The listing builds one solid part. Answer for the finished solid, in the listing's coordinates (mm). Give positions to 0.01 mm unless a question says otherwise; leave off trailing zeros. Write each loop counter-clockwise with the first axis right and the second up, starting at its lowest first coordinate (ties: lowest second). Pieces come first, ordered by that corner, then holes. Notation, with made-up numbers: M -31,22 L -6,22 A23 ccw -6,47 Z; hole C -34.75,3.25 d7. An arc over 180 degrees is marked long. Answer as a JSON object with one key per item and string values.
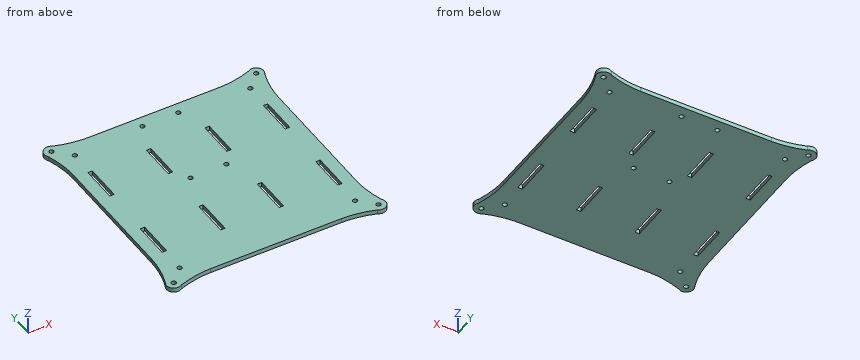
```python
from build123d import *

# Parameters (mm, degrees)
SKETCH_1_W          = 140
SKETCH_1_H          = 140
SKETCH_1_R          = 1.55
EXTRUDE_1_DEPTH     = 3
SKETCH_2_R          = 1.55
SKETCH_2_W          = 3
SKETCH_2_H          = 25
CUT_EXTRUDE_1_DEPTH = 100.040395799
SKETCH_3_R          = 3
SKETCH_3_R_2        = 1.55
EXTRUDE_2_DEPTH     = 3
FILLET_1_R          = 10
SKETCH_7_W          = 252.152927368
SKETCH_7_H          = 251.6818607
CUT_EXTRUDE_3_DEPTH = 3
SKETCH_8_R          = 1.55
CUT_EXTRUDE_4_DEPTH = 3


with BuildPart() as part:
    # 草圖1 → 填料-伸長1 (new body)
    with BuildSketch(Plane.XY):
        Rectangle(SKETCH_1_W, SKETCH_1_H)
        with Locations((-60, 60)):
            Circle(SKETCH_1_R, mode=Mode.SUBTRACT)
        with Locations((60, 60)):
            Circle(SKETCH_1_R, mode=Mode.SUBTRACT)
        with Locations((60, -60)):
            Circle(SKETCH_1_R, mode=Mode.SUBTRACT)
        with Locations((-60, -60)):
            Circle(SKETCH_1_R, mode=Mode.SUBTRACT)
    extrude(amount=EXTRUDE_1_DEPTH)

    # 草圖2 → 除料-伸長1 (cut, through all)
    with BuildSketch(Plane.XY.offset(3)):
        with Locations((-12.25, 62.5)):
            Circle(SKETCH_2_R)
        with Locations((12.25, 62.5)):
            Circle(SKETCH_2_R)
        with Locations((-12.25, 7.5)):
            Circle(SKETCH_2_R)
        with Locations((12.25, 7.5)):
            Circle(SKETCH_2_R)
        with Locations((-60, -30)):
            Rectangle(SKETCH_2_W, SKETCH_2_H)
        with Locations((-60, 30)):
            Rectangle(SKETCH_2_W, SKETCH_2_H)
        with Locations((-20, -30)):
            Rectangle(SKETCH_2_W, SKETCH_2_H)
        with Locations((-20, 30)):
            Rectangle(SKETCH_2_W, SKETCH_2_H)
        with Locations((20, 30)):
            Rectangle(SKETCH_2_W, SKETCH_2_H)
        with Locations((20, -30)):
            Rectangle(SKETCH_2_W, SKETCH_2_H)
        with Locations((60, -30)):
            Rectangle(SKETCH_2_W, SKETCH_2_H)
        with Locations((60, 30)):
            Rectangle(SKETCH_2_W, SKETCH_2_H)
    extrude(amount=-CUT_EXTRUDE_1_DEPTH, mode=Mode.SUBTRACT)

    # 草圖3 → 填料-伸長2 (add)
    # profile 1 of 4: a face of its own
    with BuildSketch(Plane.XY.offset(3)):
        with BuildLine():
            Line((-79.393398282, 100.606601718), (-48.786796564, 70))
            Line((-48.786796564, 70), (-70, 70))
            Line((-70, 70), (-70, 48.786796564))
            Line((-70, 48.786796564), (-100.606601718, 79.393398282))
            ThreePointArc((-100.606601718, 79.393398282), (-100.606601718, 100.606601718), (-79.393398282, 100.606601718))
        make_face()
        with Locations((-90, 90)):
            Circle(SKETCH_3_R, mode=Mode.SUBTRACT)
        with Locations((-81, 90)):
            Circle(SKETCH_3_R_2, mode=Mode.SUBTRACT)
        with Locations((-90, 98)):
            Circle(SKETCH_3_R_2, mode=Mode.SUBTRACT)
        with Locations(Location((-99, 90, 0), (0, 0, 180))):
            Circle(SKETCH_3_R_2, mode=Mode.SUBTRACT)
        with Locations(Location((-90, 82, 0), (0, 0, 180))):
            Circle(SKETCH_3_R_2, mode=Mode.SUBTRACT)
    # profile 2 of 4: a face of its own
    with BuildSketch(Plane.XY.offset(3)):
        with BuildLine():
            Line((48.786796564, 70), (70, 70))
            Line((70, 70), (70, 48.786796564))
            Line((70, 48.786796564), (100.606601718, 79.393398282))
            ThreePointArc((100.606601718, 79.393398282), (100.606601718, 100.606601718), (79.393398282, 100.606601718))
            Line((79.393398282, 100.606601718), (48.786796564, 70))
        make_face()
        with Locations(Location((81, 90, 0), (0, 0, 180))):
            Circle(SKETCH_3_R_2, mode=Mode.SUBTRACT)
        with Locations(Location((90, 90, 0), (0, 0, 180))):
            Circle(SKETCH_3_R, mode=Mode.SUBTRACT)
        with Locations((90, 82)):
            Circle(SKETCH_3_R_2, mode=Mode.SUBTRACT)
        with Locations(Location((90, 98, 0), (0, 0, 180))):
            Circle(SKETCH_3_R_2, mode=Mode.SUBTRACT)
        with Locations((99, 90)):
            Circle(SKETCH_3_R_2, mode=Mode.SUBTRACT)
    # profile 3 of 4: a face of its own
    with BuildSketch(Plane.XY.offset(3)):
        with BuildLine():
            Line((-48.786796564, -70), (-70, -70))
            Line((-70, -70), (-70, -48.786796564))
            Line((-70, -48.786796564), (-100.606601718, -79.393398282))
            ThreePointArc((-100.606601718, -79.393398282), (-100.606601718, -100.606601718), (-79.393398282, -100.606601718))
            Line((-79.393398282, -100.606601718), (-48.786796564, -70))
        make_face()
        with Locations((-90, -82)):
            Circle(SKETCH_3_R_2, mode=Mode.SUBTRACT)
        with Locations(Location((-90, -90, 0), (0, 0, 180))):
            Circle(SKETCH_3_R, mode=Mode.SUBTRACT)
        with Locations(Location((-81, -90, 0), (0, 0, 180))):
            Circle(SKETCH_3_R_2, mode=Mode.SUBTRACT)
        with Locations(Location((-90, -98, 0), (0, 0, 180))):
            Circle(SKETCH_3_R_2, mode=Mode.SUBTRACT)
        with Locations((-99, -90)):
            Circle(SKETCH_3_R_2, mode=Mode.SUBTRACT)
    # profile 4 of 4: a face of its own
    with BuildSketch(Plane.XY.offset(3)):
        with BuildLine():
            Line((79.393398282, -100.606601718), (48.786796564, -70))
            Line((48.786796564, -70), (70, -70))
            Line((70, -70), (70, -48.786796564))
            Line((70, -48.786796564), (100.606601718, -79.393398282))
            ThreePointArc((100.606601718, -79.393398282), (100.606601718, -100.606601718), (79.393398282, -100.606601718))
        make_face()
        with Locations(Location((90, -82, 0), (0, 0, 180))):
            Circle(SKETCH_3_R_2, mode=Mode.SUBTRACT)
        with Locations((90, -90)):
            Circle(SKETCH_3_R, mode=Mode.SUBTRACT)
        with Locations((81, -90)):
            Circle(SKETCH_3_R_2, mode=Mode.SUBTRACT)
        with Locations((90, -98)):
            Circle(SKETCH_3_R_2, mode=Mode.SUBTRACT)
        with Locations(Location((99, -90, 0), (0, 0, 180))):
            Circle(SKETCH_3_R_2, mode=Mode.SUBTRACT)
    extrude(amount=-EXTRUDE_2_DEPTH)

    # 圓角1
    fillet_1_edges = [part.edges().sort_by_distance(p)[0] for p in [
        (-48.786796564, 70, 1.5),
        (-70, 48.786796564, 1.5),
        (70, 48.786796564, 1.5),
        (48.786796564, 70, 1.5),
        (-70, -48.786796564, 1.5),
        (-48.786796564, -70, 1.5),
        (48.786796564, -70, 1.5),
        (70, -48.786796564, 1.5),
    ]]
    fillet(fillet_1_edges, radius=FILLET_1_R)

    # 草圖7 → 除料-伸長3 (cut)
    with BuildSketch(Plane.XY.offset(3)):
        Rectangle(SKETCH_7_W, SKETCH_7_H)
        with BuildLine():
            Line((-44.644660941, 70), (44.644660941, 70))
            add(Edge.make_bspline(
                [(67.004508048, 74.00337707), (55.992453544, 70.111599189), (44.644660941, 70)],
                knots=[0, 0, 0, 0.944247476, 0.944247476, 0.944247476], degree=2))
            ThreePointArc((67.004508048, 74.00337707), (73.535533906, 73.535533906), (74.00337707, 67.004508048))
            add(Edge.make_bspline(
                [(74.00337707, 67.004508048), (70.111599189, 55.992453544), (70, 44.644660941)],
                knots=[0, 0, 0, 0.944247476, 0.944247476, 0.944247476], degree=2))
            Line((70, 44.644660941), (70, -44.644660941))
            add(Edge.make_bspline(
                [(74.00337707, -67.004508048), (70.111599189, -55.992453544), (70, -44.644660941)],
                knots=[0, 0, 0, 0.944247476, 0.944247476, 0.944247476], degree=2))
            ThreePointArc((74.00337707, -67.004508048), (73.535533906, -73.535533906), (67.004508048, -74.00337707))
            add(Edge.make_bspline(
                [(67.004508048, -74.00337707), (55.992453544, -70.111599189), (44.644660941, -70)],
                knots=[0, 0, 0, 0.944247476, 0.944247476, 0.944247476], degree=2))
            Line((44.644660941, -70), (-44.644660941, -70))
            add(Edge.make_bspline(
                [(-67.004508048, -74.00337707), (-55.992453544, -70.111599189), (-44.644660941, -70)],
                knots=[0, 0, 0, 0.944247476, 0.944247476, 0.944247476], degree=2))
            ThreePointArc((-67.004508048, -74.00337707), (-73.535533906, -73.535533906), (-74.00337707, -67.004508048))
            add(Edge.make_bspline(
                [(-74.00337707, -67.004508048), (-70.111599189, -55.992453544), (-70, -44.644660941)],
                knots=[0, 0, 0, 0.944247476, 0.944247476, 0.944247476], degree=2))
            Line((-70, -44.644660941), (-70, 44.644660941))
            add(Edge.make_bspline(
                [(-74.00337707, 67.004508048), (-70.111599189, 55.992453544), (-70, 44.644660941)],
                knots=[0, 0, 0, 0.944247476, 0.944247476, 0.944247476], degree=2))
            ThreePointArc((-74.00337707, 67.004508048), (-73.535533906, 73.535533906), (-67.004508048, 74.00337707))
            add(Edge.make_bspline(
                [(-67.004508048, 74.00337707), (-55.992453544, 70.111599189), (-44.644660941, 70)],
                knots=[0, 0, 0, 0.944247476, 0.944247476, 0.944247476], degree=2))
        make_face(mode=Mode.SUBTRACT)
    extrude(amount=-CUT_EXTRUDE_3_DEPTH, mode=Mode.SUBTRACT)

    # 草圖8 → 除料-伸長4 (cut)
    with BuildSketch(Plane.XY.offset(3)):
        with Locations((-70, 70)):
            Circle(SKETCH_8_R)
        with Locations((70, 70)):
            Circle(SKETCH_8_R)
        with Locations((70, -70)):
            Circle(SKETCH_8_R)
        with Locations((-70, -70)):
            Circle(SKETCH_8_R)
    extrude(amount=-CUT_EXTRUDE_4_DEPTH, mode=Mode.SUBTRACT)


solid = part.part
```
1. A cutting plane is placed at B-B, the plane x = -16. Give the vertices of the cut face in (y, z).
Verdict:
{"outline": "M -70,0 L 70,0 L 70,3 L -70,3 Z"}
2. A cutting plane is placed at C-C, the plane z = 1.15. Count the separate pieces of the cut face and the enclosed holes in it, plus the area to 3 significant figures.
Verdict:
{"separate pieces": "1", "enclosed holes": "20", "area": "19,300 mm2"}
3. A cutting plane is placed at A-A, the plane y = 21. Give the vertices of the cut face in (x, z), plus the area to 3 significant figures.
Verdict:
{"outline": "M -70,0 L -61.5,0 L -61.5,3 L -70,3 Z; M -58.5,0 L -21.5,0 L -21.5,3 L -58.5,3 Z; M -18.5,0 L 18.5,0 L 18.5,3 L -18.5,3 Z; M 21.5,0 L 58.5,0 L 58.5,3 L 21.5,3 Z; M 61.5,0 L 70,0 L 70,3 L 61.5,3 Z", "area": "384 mm2"}
4. Consider line 1 along Y through (x, z) = (-20, 2.1); line 2 along X through (y, z) = (29, 0.7); line 3 along Y through (x, z) = (12.25, 2). Determine where each line is inside the solid, lowest interval first.
Verdict:
{"line 1": "y = -70 to -42.5, -17.5 to 17.5, 42.5 to 70", "line 2": "x = -70 to -61.5, -58.5 to -21.5, -18.5 to 18.5, 21.5 to 58.5, 61.5 to 70", "line 3": "y = -70 to 5.95, 9.05 to 60.95, 64.05 to 70"}
5. Flat-ended cylindrical pins translate along their axes: pin 1 (1.5 mm diameter, centred on y = -33, z = 1, fed in from -X); pin 2 (1.5 mm diameter, centred on y = 32.5, z = 1.5, fed in from +X); pin 3 (1.9 mm diameter, centred on x = 12.25, y = 62.5, fed in from -Z); pin 4 (1.5 mm diameter, centred on x = 19.5, z = 1, fed in from +Y). Find the tip coordinate at first contact, or state that the pin passes through.
Verdict:
{"pin 1": "stops at x = -70", "pin 2": "stops at x = 70", "pin 3": "passes through", "pin 4": "stops at y = 70"}
